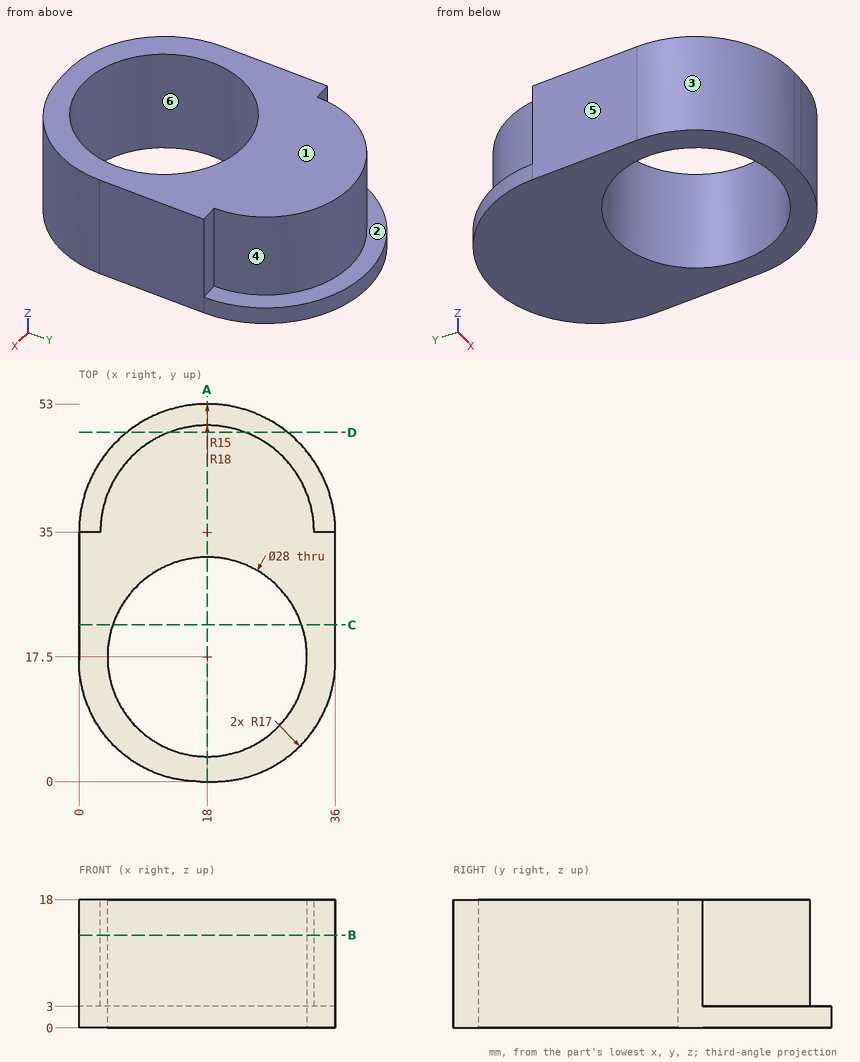
Job drawing, mm, ordinate dimensions from the low corner. One solid piece. A direction names the side the tool comes from. Give positions to 0.01 mm unless a question says otherwise; leave off trailing zeros. Order: outer loops, then holes, each group sorted by start corner. A loop starts at its lowest first (then second) coordinate and runs counter-clockwise, first axis right, second up. Notation, with made-up numbers: (88.5, -2) - (113.5, -2) arc R17 cw to (113.5, 19) - close; hole circle Ø8 at (22, -30.75). An arc over 180 degrees is marked (long way). Return JSON: item names as keys, results as strings.
1) Probe line 1 (Y direction, x = 18, z = 5.25); line 2 (X direction, y = 12.5, z = 5.5); line 3 (Z direction, x = 34.5, y = 37). List the from-to ranges inside material, lowest first. Write a range as from..to.
Geometry says:
{"line 1": "0..3.5, 31.5..50", "line 2": "0.61..4.92, 31.08..35.39", "line 3": "0..3"}
2) Cut at C-C, the plane y = 22. Give the cut face in (x, z), plus the area to 3 significant figures.
Geometry says:
{"outline": "(0, 0) - (4.74, 0) - (4.74, 18) - (0, 18) - close; (31.26, 0) - (36, 0) - (36, 18) - (31.26, 18) - close", "area": "171 mm²"}
3) Flat gauge pins, fed straight in: P1, Ø2, axis at x = 22, z = 10, coming from the +Y side; P2, Ø10, axis at x = 27, z = 2.5, coming from the +Y side; P3, Ø2, axis at x = 30, z = 6, coming from the -Y side. Where does each tip first touch, or does it go through?
Geometry says:
{"P1": "y = 49.7", "P2": "y = 52.55", "P3": "y = 3.25"}
4) 3-axis set-ups, long thin cutter, end or side, ignore diameter. For the marked faces 1 and 2: which of +Z, -Z, +X, -X, +Y, -Y reach the whole face in a straight line?
Geometry says:
{"face 1": "+Z, +X, -X, +Y, -Y", "face 2": "+Z, +Y"}
5) Cut at B-B, the plane z = 13. Give the cut face in (x, y), plus the area to 3 significant figures.
Geometry says:
{"outline": "(0, 17) arc R17 ccw to (17, 0) - (19, 0) arc R17 ccw to (36, 17) - (36, 35) - (33, 35) arc R15 ccw to (3, 35) - (0, 35) - close; hole circle Ø28 at (18, 17.5)", "area": "874 mm²"}
6) Cut at A-A, the plane x = 18. Give the cut face in (y, z), plus the area to 3 significant figures.
Geometry says:
{"outline": "(0, 0) - (3.5, 0) - (3.5, 18) - (0, 18) - close; (31.5, 0) - (53, 0) - (53, 3) - (50, 3) - (50, 18) - (31.5, 18) - close", "area": "405 mm²"}
7) Cut at D-D, the plane y = 49. Give the cut face in (x, z).
Geometry says:
{"outline": "(6.69, 0) - (29.31, 0) - (29.31, 3) - (23.39, 3) - (23.39, 18) - (12.61, 18) - (12.61, 3) - (6.69, 3) - close"}
8) Pull direction Y, two halves, no side cores. Call the marked faces 3, 4, 5 and 6: pulls with the +Y half, pulls with the -Y half, needs draft (parallel to the pull), parting line crosses it, or undercut.
Geometry says:
{"face 3": "pulls with the -Y half", "face 4": "pulls with the +Y half", "face 5": "needs draft", "face 6": "undercut"}
